Build history of the part. All positions in model axes, mm. A direction names the side the tool comes from. Give positions to 0.01 mm unless a question says otherwise; leave off trailing zeros. Loops run counter-clockwise (first coordinate to the right, second up) from the corner with the lowest first, then second, coordinate; pieces in that order, holes last. Notation, with made-up numbers: (82.25, 36.25) -> (87.25, 36.25) arc R24 ccw to (87.25, 59.25) -> close; hole circle Ø9 at (42.25, 10). An arc over 180 degrees is marked (long way). Answer as a JSON object with one key per item and string values. Group by question number.
from build123d import *

# Parameters (mm, degrees)
SKETCH_1_W               = 12
SKETCH_1_H               = 10
SKETCH_1_R               = 1.5
EXTRUDE_1_DEPTH          = 1
SKETCH_4_R               = 1.5
SKETCH_4_R_2             = 0.9
EXTRUDE_2_DEPTH          = 3.5
SKETCH_5_R               = 0.5
EXTRUDE_3_DEPTH          = 1
SKETCH_6_R               = 1.5
SKETCH_6_R_2             = 0.9
EXTRUDE_4_DEPTH          = 2.5
SKETCH_7_W               = 12
SKETCH_7_H               = 10
SKETCH_7_R               = 0.532937176
SKETCH_7_R_2             = 0.5
EXTRUDE_5_DEPTH          = 1
FILLET_1_R               = 1
HOLE_WIZARD_1_AT_2_COUNT = 2
HOLE_WIZARD_1_AT_2_PITCH = 8.602325267
HOLE_WIZARD_M1_6_1_D     = 1.25
HOLE_WIZARD_M1_6_1_DEPTH = 1
SKETCH_12_R              = 2
SKETCH_12_R_2            = 1.5
EXTRUDE_6_DEPTH          = 0.7
FILLET_2_R               = 0.3


with BuildPart() as part:
    # 草图1 → 凸台-拉伸1 (new body)
    with BuildSketch(Plane.XY):
        Rectangle(SKETCH_1_W, SKETCH_1_H)
        Circle(SKETCH_1_R, mode=Mode.SUBTRACT)
    extrude(amount=EXTRUDE_1_DEPTH)

    # 草图4 → 凸台-拉伸2 (add)
    with BuildSketch(Plane(origin=(0, 0, 0), x_dir=(-1, 0, 0), z_dir=(0, 0, -1))):
        with Locations((-3.5, 2.5)):
            Circle(SKETCH_4_R)
        with Locations((-3.5, 2.5)):
            Circle(SKETCH_4_R_2, mode=Mode.SUBTRACT)
        with Locations((3.5, -2.5)):
            Circle(SKETCH_4_R)
        with Locations((3.5, -2.5)):
            Circle(SKETCH_4_R_2, mode=Mode.SUBTRACT)
    extrude(amount=EXTRUDE_2_DEPTH)

    # 草图5 → 凸台-拉伸3 (add)
    with BuildSketch(Plane(origin=(0, 0, -3.5), x_dir=(-1, 0, 0), z_dir=(0, 0, -1))):
        Polygon((-6, -5), (-6, 5), (1, 5), (1, 0), (6, 0), (6, -5), align=None)
        with Locations((-3, -3)):
            Circle(SKETCH_5_R, mode=Mode.SUBTRACT)
        Circle(SKETCH_5_R, mode=Mode.SUBTRACT)
    extrude(amount=EXTRUDE_3_DEPTH)

    # 草图6 → 凸台-拉伸4 (add)
    with BuildSketch(Plane(origin=(0, 0, -4.5), x_dir=(-1, 0, 0), z_dir=(0, 0, -1))):
        with Locations((3.5, -2.5)):
            Circle(SKETCH_6_R)
        with Locations((3.5, -2.5)):
            Circle(SKETCH_6_R_2, mode=Mode.SUBTRACT)
        with Locations((-3.5, 2.5)):
            Circle(SKETCH_6_R)
        with Locations((-3.5, 2.5)):
            Circle(SKETCH_6_R_2, mode=Mode.SUBTRACT)
    extrude(amount=EXTRUDE_4_DEPTH)

    # 草图7 → 凸台-拉伸5 (add)
    with BuildSketch(Plane(origin=(0, 0, -7), x_dir=(-1, 0, 0), z_dir=(0, 0, -1))):
        Rectangle(SKETCH_7_W, SKETCH_7_H)
        Circle(SKETCH_7_R, mode=Mode.SUBTRACT)
        with Locations((3, 2.5)):
            Circle(SKETCH_7_R_2, mode=Mode.SUBTRACT)
    extrude(amount=EXTRUDE_5_DEPTH)

    # 圆角1
    fillet_1_edges = [part.edges().sort_by_distance(p)[0] for p in [
        (6, -5, -4),
        (-6, -5, -4),
        (-6, 0, -4),
        (-1, 0, -4),
        (-1, 5, -4),
        (6, 5, -4),
        (-6, 5, -7.5),
        (6, 5, -7.5),
        (6, -5, -7.5),
        (-6, -5, -7.5),
        (6, -5, 0.5),
        (-6, -5, 0.5),
        (-6, 5, 0.5),
        (6, 5, 0.5),
    ]]
    fillet(fillet_1_edges, radius=FILLET_1_R)

    # 草图8 → 打孔尺寸根据开槽半沉头木螺钉的类型1 (revolve, cut)
    with BuildSketch(Plane(origin=(3.5, 2.5, 1), x_dir=(0, -1, 0), z_dir=(1, 0, 0))):
        Polygon((0, 0), (0, 1), (0.9, 1), (0.9, 0.85), (1.75, 0), align=None)
    hole_wizard_1 = revolve(axis=Axis((3.5, 2.5, 7.35), (0, 0, -1)), mode=Mode.SUBTRACT)

    # 打孔尺寸根据开槽半沉头木螺钉的类型1 at 2: 打孔尺寸根据开槽半沉头木螺钉的类型1 ×2
    with Locations(*[Vector(-0.813733471, -0.581238194, 0) * (i * HOLE_WIZARD_1_AT_2_PITCH) for i in range(1, HOLE_WIZARD_1_AT_2_COUNT)]):
        add(hole_wizard_1, mode=Mode.SUBTRACT)

    # M1.6 螺纹孔1
    with Locations(Plane.XY.offset(1)):
        with Locations((4.5, 0), (-4.5, 0)):
            Hole(HOLE_WIZARD_M1_6_1_D / 2, depth=HOLE_WIZARD_M1_6_1_DEPTH)

    # 草图12 → 凸台-拉伸6 (add)
    with BuildSketch(Plane.XY.offset(1)):
        Circle(SKETCH_12_R)
        Circle(SKETCH_12_R_2, mode=Mode.SUBTRACT)
    extrude(amount=EXTRUDE_6_DEPTH)

    # 圆角2
    fillet_2_edges = [part.edges().sort_by_distance(p)[0] for p in [
        (-2, 0, 1.7),
    ]]
    fillet(fillet_2_edges, radius=FILLET_2_R)


solid = part.part
(1) Saw through at C-C on z = 1.25. List the corners of the cut face in (x, y), plus the area to 3 significant figures.
(2) Pull direction Y, two halves, no side cores. Call faces 4 (the cylindrical face through (0.532, 0.023, -7.493)), 5 (the flat face through (0, -5, -4)), 6 (the cylindrical face through (2.114, 1.925, -5.732)): pulls with the +Y half, pulls with the -Y half, needs draft (parallel to the pull), parting line crosses it, or undercut.
(3) Pin check, flat tips, straight feed: pin 1 (0.9 mm diameter, centred on x = 3.5, y = 2.5, fed in from +Z); pin 2 (1.6 mm diameter, centred on x = -4.5, y = 0, fed in from +Z); pin 3 (0.9 mm diameter, centred on x = 3.5, y = 3, fed in from +Z). Stop position of each tip, or through.
(4) Probe line 1 along Z through (x, y) = (0.5, -4); line 2 along Y through (x, z) = (0, -7.5); line 3 along Z through (x, y) = (-2.5, 4.5). List the from-to ranges inside material, lowest first. Write a range as [from, to].
(5) Saw through at B-B on z = -2.5. List the corners of the cut face in (x, y).
(6) Saw through at A-A on y = 2.5. Give the number of separate pieces and of enclosed holes in the cut face, plus the area to 3 significant figures.
(7) 3-axis set-ups, long thin cutter, end or side, ignore diameter. For faces 1 (the cylindrical face through (-5.715, -4.699, 0.507)), 2 (the cylindrical face through (2.114, 1.925, -1.726)), 3 (the cylindrical face through (-1.5, 0.07, 0.84)): which of +Z, -Z, +X, -X, +Y, -Y reach the whole face in a straight line?
Calculated:
{
 "1": {"outline": "circle Ø4 at (0, 0); hole circle Ø3 at (0, 0)", "area": "5.50 mm^2"},
 "2": {"face 4": "undercut", "face 5": "pulls with the -Y half", "face 6": "parting line crosses it"},
 "3": {"pin 1": "stops at z = -3.5", "pin 2": "stops at z = 1", "pin 3": "stops at z = 0.2"},
 "4": {"line 1": "z = [-8, -7], [-4.5, -3.5], [0, 1]", "line 2": "y = [-5, -0.53], [0.53, 5]", "line 3": "z = [-8, -7], [0, 1]"},
 "5": {"outline": "circle Ø3 at (-3.5, -2.5); circle Ø3 at (3.5, 2.5); hole circle Ø1.8 at (-3.5, -2.5); hole circle Ø1.8 at (3.5, 2.5)"},
 "6": {"separate pieces": "2", "enclosed holes": "1", "area": "34.7 mm^2"},
 "7": {"face 1": "+Z, -Z, -X, -Y", "face 2": "none", "face 3": "+Z"}
}
